```python
from build123d import *

# Parameters (mm, degrees)
SKETCH_1_W               = 270
SKETCH_1_H               = 79
EXTRUDE_1_DEPTH          = 2.6
SKETCH_2_W               = 200
SKETCH_2_H               = 60
CUT_EXTRUDE_1_DEPTH      = 141.684078701
FILLET_1_SIZE            = 5
FILLET_1_SIZE_2          = 1.8
SKETCH_3_W               = 5
SKETCH_3_H               = 2
CUT_EXTRUDE_2_DEPTH      = 141.684078827
MIRROR_2_COPY_1_SKETCH_W = 5
MIRROR_2_COPY_1_SKETCH_H = 2
MIRROR_2_COPY_1_DEPTH    = 141.684078827


with BuildPart() as part:
    # 草图1 → 凸台-拉伸1 (new body)
    with BuildSketch(Plane.XY):
        Rectangle(SKETCH_1_W, SKETCH_1_H)
    extrude(amount=EXTRUDE_1_DEPTH)

    # 草图2 → 切除-拉伸1 (cut, through all)
    with BuildSketch(Plane.XY.offset(2.6)):
        Rectangle(SKETCH_2_W, SKETCH_2_H)
    extrude(amount=-CUT_EXTRUDE_1_DEPTH, mode=Mode.SUBTRACT)

    # 圆角1
    # an asymmetric fillet: 5, 1.8 mm, written as the material it takes off along each edge
    with BuildSketch(Plane(origin=(135, -39.5, -12.5), x_dir=(0, 1, 0), z_dir=(0, 0, 1))) as fillet_1_piece_1:
        with BuildLine():
            Bezier((FILLET_1_SIZE, 0), (0, 0), (0, FILLET_1_SIZE_2), weights=[1, 0.707106781, 1])
            Line((0, FILLET_1_SIZE_2), (0, 0))
            Line((0, 0), (FILLET_1_SIZE, 0))
        make_face()
    extrude(amount=27.6, mode=Mode.SUBTRACT)
    with BuildSketch(Plane(origin=(135, 39.5, -12.5), x_dir=(-1, 0, 0), z_dir=(0, 0, 1))) as fillet_1_piece_2:
        with BuildLine():
            Bezier((FILLET_1_SIZE_2, 0), (0, 0), (0, FILLET_1_SIZE), weights=[1, 0.707106781, 1])
            Line((0, FILLET_1_SIZE), (0, 0))
            Line((0, 0), (FILLET_1_SIZE_2, 0))
        make_face()
    extrude(amount=27.6, mode=Mode.SUBTRACT)
    with BuildSketch(Plane(origin=(-135, -39.5, -12.5), x_dir=(0, 1, 0), z_dir=(0, 0, 1))) as fillet_1_piece_3:
        with BuildLine():
            Bezier((FILLET_1_SIZE, 0), (0, 0), (0, -FILLET_1_SIZE_2), weights=[1, 0.707106781, 1])
            Line((0, -FILLET_1_SIZE_2), (0, 0))
            Line((0, 0), (FILLET_1_SIZE, 0))
        make_face()
    extrude(amount=27.6, mode=Mode.SUBTRACT)
    with BuildSketch(Plane(origin=(-135, 39.5, -12.5), x_dir=(1, 0, 0), z_dir=(0, 0, 1))) as fillet_1_piece_4:
        with BuildLine():
            Bezier((FILLET_1_SIZE_2, 0), (0, 0), (0, -FILLET_1_SIZE), weights=[1, 0.707106781, 1])
            Line((0, -FILLET_1_SIZE), (0, 0))
            Line((0, 0), (FILLET_1_SIZE_2, 0))
        make_face()
    extrude(amount=27.6, mode=Mode.SUBTRACT)

    # 草图3 → 切除-拉伸2 (cut, through all)
    with BuildSketch(Plane.XY.offset(2.6)):
        with Locations((-124.5, 38.5)):
            Rectangle(SKETCH_3_W, SKETCH_3_H)
    cut_extrude_2 = extrude(amount=-CUT_EXTRUDE_2_DEPTH, mode=Mode.SUBTRACT)

    # 镜向1: 切除-拉伸2 across plane
    add(cut_extrude_2.mirror(Plane.ZX), mode=Mode.SUBTRACT)

    # 镜向2: 切除-拉伸2 across plane
    add(cut_extrude_2.mirror(Plane(origin=(0, 0, 0), x_dir=(0, 0, 1), z_dir=(1, 0, 0))), mode=Mode.SUBTRACT)

    # 镜向2 copy 1 sketch → 镜向2 copy 1 (cut, through all)
    with BuildSketch(Plane(origin=(0, 0, 2.6), x_dir=(-1, 0, 0), z_dir=(0, 0, 1))):
        with Locations((-124.5, 38.5)):
            Rectangle(MIRROR_2_COPY_1_SKETCH_W, MIRROR_2_COPY_1_SKETCH_H)
    extrude(amount=-MIRROR_2_COPY_1_DEPTH, mode=Mode.SUBTRACT)


solid = part.part
```
Verification items for the finished model (mm, model axes). Coordinates: 2 decimals unless noted, no trailing zeros. Write each loop counter-clockwise with the first axis right and the second up, starting at its lowest first coordinate (ties: lowest second). Pieces come first, ordered by that corner, then holes. Notation, with made-up numbers: (44, 67.5) - (84, 67.5) arc R23 ccw to (84, 102.5) - close; hole circle Ø6 at (84, 22.5). An arc over 180 degrees is marked (long way). Write item = value, one per line.
Q1. Go/stop test with flat-tipped pins: pin 1 Ø0.6 at (y, z) = (-38, 1) entering from -X; pin 2 Ø0.6 at (y, z) = (38.5, 1.5) entering from -X; pin 3 Ø1.3 at (x, z) = (-124, 2) entering from -Y. Record where each tip stops, or that it passes through.
Answer:
pin_1 = -134.58
pin_2 = -134.41
pin_3 = -37.5
Q2. Cross-section at A-A (x = 87.5). Enter the section's corners in (y, z), plus the area to 3 significant figures.
Answer:
outline = (-39.5, 0) - (-30, 0) - (-30, 2.6) - (-39.5, 2.6) - close; (30, 0) - (39.5, 0) - (39.5, 2.6) - (30, 2.6) - close
area = 49.4 mm²
Q3. Cross-section at B-B (y = -1). Enter the section's corners in (x, z).
Answer:
outline = (-135, 0) - (-100, 0) - (-100, 2.6) - (-135, 2.6) - close; (100, 0) - (135, 0) - (135, 2.6) - (100, 2.6) - close
Q4. Material ranges on L1, parallel to X at y = 1, z = 2.45; L2, parallel to Y at x = -1, z = 2; L3, parallel to X at y = 35.5, z = 0.9, recorded low to high. Write a range as from..to.
Answer:
L1 = -135..-100, 100..135
L2 = -39.5..-30, 30..39.5
L3 = -134.96..134.96
